Autodesk Inventor part; units mm, degrees
ref_plane "YZ Plane" through (0, 0, 0) normal (1, 0, 0) x (0, 1, 0)
ref_plane "XZ Plane" through (0, 0, 0) normal (0, 1, 0) x (-1, 0, 0)
ref_plane "XY Plane" through (0, 0, 0) normal (0, 0, 1) x (1, 0, 0)
sketch "Sketch1" plane through (0, 0, 0) normal (0, 1, 0) x (-1, 0, 0)
  line L0 (4.5, 1.988) -> (3.1372, -1.1754)
  line L1 (3.1372, -1.1754) -> (-0.0634, -2.4486)
  line L2 (-0.0634, -2.4486) -> (-3.2268, -1.0858)
  line L3 (-3.2268, -1.0858) -> (-4.5, 2.1147)
  line L4 (-4.5, 2.1147) -> (-3.1372, 5.2782)
  line L5 (-3.1372, 5.2782) -> (0.0634, 6.5514)
  line L6 (0.0634, 6.5514) -> (3.2268, 5.1885)
  line L7 (3.2268, 5.1885) -> (4.5, 1.988)
  point P0 (0, 0)
  point P1 (0, 2.0514)
  dimension "d0" = 9
extrude "Extrusion1" add sketch "Sketch1" along normal blind 5
sketch "Sketch2" plane through (0, 5, 0) normal (0, 1, 0) x (1, 0, 0)
  line L0 (-3.1372, 1.1754) -> (-4.5, -1.988)
  line L1 (-4.5, -1.988) -> (-3.1372, 1.1754)
  line L2 (0.0634, 2.4486) -> (-3.1372, 1.1754)
  line L3 (-3.1372, 1.1754) -> (0.0634, 2.4486)
  line L4 (3.2268, 1.0858) -> (0.0634, 2.4486)
  line L5 (0.0634, 2.4486) -> (3.2268, 1.0858)
  line L6 (4.5, -2.1147) -> (3.2268, 1.0858)
  line L7 (3.2268, 1.0858) -> (4.5, -2.1147)
  line L8 (4.5, -2.1147) -> (-4.5, -1.988)
  point P0 (0, 0)
extrude "Extrusion2" cut sketch "Sketch2" against normal blind 2.5
sketch "Sketch3" plane through (0, 2.5, 0) normal (0, 1, 0) x (1, 0, 0)
  line L0 (-3.1372, 1.1754) -> (0.0634, 2.4486)
  circle A0 centre (-3.1372, 1.1754) radius 1
  circle A1 centre (0.0634, 2.4486) radius 1
  line L1 (0.0634, 2.4486) -> (3.2268, 1.0858)
  circle A2 centre (3.2268, 1.0858) radius 1
  point P0 (0, 0)
  dimension "d5" = 2
  dimension "d6" = 2
  dimension "d7" = 2
extrude "Extrusion3" cut sketch "Sketch3" against normal blind 1
sketch "Sketch4" plane through (0, 5, 0) normal (0, 1, 0) x (1, 0, 0)
  line L0 (-3.2268, -5.1885) -> (-4.5, -1.988)
  circle A0 centre (-3.2268, -5.1885) radius 1
  line L1 (-0.0634, -6.5514) -> (-3.2268, -5.1885)
  circle A1 centre (-0.0634, -6.5514) radius 1
  line L2 (4.5, -2.1147) -> (3.1372, -5.2782)
  circle A2 centre (3.1372, -5.2782) radius 1
  point P0 (0, 0)
  dimension "d10" = 2
  dimension "d11" = 2
  dimension "d12" = 2
extrude "Extrusion4" cut sketch "Sketch4" against normal blind 1
sketch "Sketch5" plane through (0, 0, 0) normal (0, -1, 0) x (1, 0, 0)
  line L0 (4.5, 2.1147) -> (-4.5, 1.988)
  circle A0 centre (0, 2.0514) radius 0.875
  point P0 (0, 0)
  dimension "d15" = 1.75
extrude "Extrusion5" cut sketch "Sketch5" against normal through all
sketch "Sketch6" plane through (0, 2.5, 0) normal (0, 1, 0) x (1, 0, 0)
  arc A0 (0.8749, -2.0637) -> (-0.8749, -2.039) centre (0, -2.0514) ccw
  circle A1 centre (0, -2.0514) radius 2
  point P0 (0, 0)
  dimension "d18" = 4
extrude "Extrusion6" add sketch "Sketch6" along normal blind 35
sketch "Sketch7" plane through (0, 2.5, 2.0514) normal (0, -1, 0) x (1, 0, 0)
  circle A0 centre (0, 0) radius 0.875
  point P0 (0, -2.0514)
  dimension "d23" = 1.75
extrude "Extrusion7" cut sketch "Sketch7" against normal blind 31
fillet "Fillet1" radius 2 1 edges at (-2, 37.5, 2.0514)
properties part number "driver_handle"
The model under review builds one solid part; all positions refer to its coordinate system, in mm. A direction names the side the tool comes from. Give positions to 0.01 mm unless a question says otherwise; leave off trailing zeros. Loops run counter-clockwise (first coordinate to the right, second up) from the corner with the lowest first, then second, coordinate; pieces in that order, holes last. Notation, with made-up numbers: (38.5, 49) -> (55.5, 49) arc R31 ccw to (55.5, 83) -> close; hole circle Ø7 at (55, -7). An arc over 180 degrees is marked (long way). Answer as a JSON object with one key per item and string values. Group by question number.
Q1. Tool access review of faces 4 (the cylindrical face through (0.03, 2.01, -1.45)), 5 (the flat face through (3.83, 2.46, 3.67)), 6 (the cylindrical face through (-2.45, 2.01, -0.45)), 7 (the flat face through (-3.98, 1.23, 0.78)), 8 (the flat face through (0, 4, 6)): name each direction out of +Z, -Z, +X, -X, +Y, -Y from which nothing blocks a thin tool from reaching the whole face with its end or side.
Q2. Wall thickness on line 1 along Z through (x, y) = (0, 23.5); line 2 along X through (y, z) = (24, 2); line 3 along Y through (x, z) = (-1.5, -1.5): over which ranges is each line inside the solid? List them lowest first.
Q3. Take a section at C-C (y = 24). Write out the cut boundary in (x, z) (3 decimals), plus the area to 3 significant figures.
Q4. Draft analysis for pull direction X (two halves, no side actions). For faces 1 (the flat face through (0, 5, 5)), 2 (the cylindrical face through (2.5, 2, -0.4)), 3 (the flat face through (1.62, 0.95, -1.78)), state which applies: pulls with the +X half, pulls with the -X half, needs draft (parallel to the pull), parting line crosses it, or undercut.
Q5. Take a section at B-B (z = 3.25). Write out the cut boundary in (x, y).
Q6. Take a section at A-A (x = 0.5). Write out the cut boundary in (y, z), plus the area to 3 significant figures.
Q7. Insertion check: pin 1 (1 mm diameter, centred on x = 2.5, z = 4, fed in from +Y); pin 2 (4.5 mm diameter, centred on x = 0.5, z = -0.5, fed in from +Y); pin 3 (1.6 mm diameter, centred on x = 0, z = 2.05, fed in from -Y). Each pin has a flat end and moves straight along its axis. Give the tip position at first contact, or say it passes through.
Q8. Take a section at D-D (z = 1.5). Write out the cut boundary in (x, y).
Answer below:
{
 "1": {"face 4": "-Z, +Y", "face 5": "+Z, +X, +Y, -Y", "face 6": "+Y", "face 7": "-Z, -X, +Y, -Y", "face 8": "+Z, +Y"},
 "2": {"line 1": "z = 0.05 to 1.18, 2.93 to 4.05", "line 2": "x = -2 to -0.87, 0.87 to 2", "line 3": "y = 0 to 2.5"},
 "3": {"outline": "circle Ø4 at (0, 2.051); hole circle Ø1.75 at (0, 2.051)", "area": "10.2 mm2"},
 "4": {"face 1": "needs draft", "face 2": "undercut", "face 3": "pulls with the +X half"},
 "5": {"outline": "(-4, 0) -> (4.01, 0) -> (4.01, 5) -> (1.6, 5) -> (1.6, 35.5) arc R1.6 ccw to (-1.6, 35.5) -> (-1.6, 5) -> (-4, 5) -> close"},
 "6": {"outline": "(0, -2.26) -> (1.5, -2.26) -> (1.5, -1.55) -> (2.5, -1.55) -> (2.5, 0.11) -> (35.5, 0.11) arc R1.94 ccw to (35.5, 3.99) -> (5, 3.99) -> (5, 5.73) -> (4, 5.73) -> (4, 6.33) -> (0, 6.33) -> (0, 2.77) -> (33.5, 2.77) -> (33.5, 1.33) -> (0, 1.33) -> close", "area": "112 mm2"},
 "7": {"pin 1": "stops at y = 5", "pin 2": "stops at y = 37.47", "pin 3": "stops at y = 33.5"},
 "8": {"outline": "(-4.29, 0) -> (-0.68, 0) -> (-0.68, 33.5) -> (0.68, 33.5) -> (0.68, 0) -> (4.26, 0) -> (4.26, 2.5) -> (1.92, 2.5) -> (1.92, 35.5) arc R1.92 ccw to (-1.92, 35.5) -> (-1.92, 2.5) -> (-4.29, 2.5) -> close"}
}
